Read the model definition and answer for the solid it produces. Units are mm, in the model's axes. A direction names the side the tool comes from. Give positions to 0.01 mm unless a question says otherwise; leave off trailing zeros. Write each loop counter-clockwise with the first axis right and the second up, starting at its lowest first coordinate (ties: lowest second). Pieces come first, ordered by that corner, then holes. Notation, with made-up numbers: (-32.5, 16) - (-26.5, 16) arc R32 cw to (-26.5, 46) - close; hole circle Ø7 at (-9.75, 49.5). An arc over 180 degrees is marked (long way). Answer as a JSON object with one key per item and string values. Group by question number.
```python
from build123d import *

# Parameters (mm, degrees)
SKETCH1_W           = 62.8
SKETCH1_H           = 46
SKETCH1_R           = 1.4
SKETCH1_R_2         = 15
BOSS_EXTRUDE1_DEPTH = 6
SKETCH2_W           = 8.5
SKETCH2_H           = 15
CUT_EXTRUDE1_DEPTH  = 41.459856648
FILLET1_R           = 3.1
CUT_EXTRUDE2_DEPTH  = 41.459856648


with BuildPart() as part:
    # Sketch1 → Boss-Extrude1 (new body)
    with BuildSketch(Plane(origin=(0, 0, 0), x_dir=(1, 0, 0), z_dir=(0, 1, 0))):
        with Locations((0, -1.8)):
            Rectangle(SKETCH1_W, SKETCH1_H)
        with Locations(Location((-28.3, -1.4, 0), (0, 0, 270))):
            Circle(SKETCH1_R, mode=Mode.SUBTRACT)
        with Locations(Location((28.3, 3.1, 0), (0, 0, 270))):
            Circle(SKETCH1_R, mode=Mode.SUBTRACT)
        with Locations(Location((-0.6, -0.8, 0), (0, 0, 270))):
            Circle(SKETCH1_R_2, mode=Mode.SUBTRACT)
    extrude(amount=BOSS_EXTRUDE1_DEPTH)

    # Sketch2 → Cut-Extrude1 (cut, through all)
    with BuildSketch(Plane(origin=(0, 6, 0), x_dir=(1, 0, 0), z_dir=(0, 1, 0))):
        with Locations((27.15, 13.7)):
            Rectangle(SKETCH2_W, SKETCH2_H)
        with BuildLine():
            Line((14.4, -24.8), (31.4, -24.8))
            Line((31.4, -24.8), (31.4, 0))
            Line((31.4, 0), (22.9, 0))
            ThreePointArc((22.9, 0), (20.676259907, -10.31612815), (14.4, -18.8))
            Line((14.4, -18.8), (14.4, -24.8))
        make_face()
        with BuildLine():
            Line((-17.4, -24.8), (-17.4, -16.8))
            ThreePointArc((-17.4, -16.8), (-21.820028515, -11.342696837), (-23.4, -4.5))
            Line((-23.4, -4.5), (-31.4, -4.5))
            Line((-31.4, -4.5), (-31.4, -24.8))
            Line((-31.4, -24.8), (-17.4, -24.8))
        make_face()
        with BuildLine():
            Line((-20.1, 21.2), (-20.1, 11.2))
            ThreePointArc((-20.1, 11.2), (-22.551509918, 6.728419235), (-23.4, 1.7))
            Line((-23.4, 1.7), (-31.4, 1.7))
            Line((-31.4, 1.7), (-31.4, 21.2))
            Line((-31.4, 21.2), (-20.1, 21.2))
        make_face()
    extrude(amount=-CUT_EXTRUDE1_DEPTH, mode=Mode.SUBTRACT)

    # Fillet1
    fillet1_edges = [part.edges().sort_by_distance(p)[0] for p in [
        (-31.4, 3, 4.5),
        (-31.4, 3, -1.7),
        (31.4, 3, -6.2),
        (31.4, 3, 0),
    ]]
    fillet(fillet1_edges, radius=FILLET1_R - 0.0001)  # a hair under: the kernel refuses the full size

    # Sketch3 → Cut-Extrude2 (cut, through all)
    with BuildSketch(Plane(origin=(0, 6, 0), x_dir=(1, 0, 0), z_dir=(0, 1, 0))):
        with BuildLine():
            Line((28.3, 0), (24.9, 0))
            Line((24.9, 0), (24.9, 6.2))
            Line((24.9, 6.2), (28.3, 6.2))
            ThreePointArc((28.3, 6.2), (30.492031022, 5.292031022), (31.4, 3.1))
            ThreePointArc((31.4, 3.1), (30.492031022, 0.907968978), (28.3, 0))
        make_face()
        with BuildLine():
            Line((-25.1, -4.5), (-28.3, -4.5))
            ThreePointArc((-28.3, -4.5), (-30.492031022, -3.592031022), (-31.4, -1.4))
            ThreePointArc((-31.4, -1.4), (-30.492031022, 0.792031022), (-28.3, 1.7))
            Line((-28.3, 1.7), (-25.1, 1.7))
            Line((-25.1, 1.7), (-25.1, -4.5))
        make_face()
    extrude(amount=-CUT_EXTRUDE2_DEPTH, mode=Mode.SUBTRACT)


with BuildPart() as cut_extrude2_kept_piece:
    # of the separate pieces the step leaves, the one the design keeps (cut_extrude2_pieces_kept)
    add(part.part.solids().sort_by_distance((-23.4, 0, 4.5))[0])


solid = cut_extrude2_kept_piece.part
```
1) Find section D-D, the plane x = -21. Write down the section's boundary in (y, z), and give its area (3 significant figures).
2) For a pull along Z with two mould halves and no side action, classify faces 5 (the cylindrical face through (-22.528, 3.042, -6.796)), 6 (the flat face through (11, 6, 12)), 7 (the cylindrical face through (-6.345, 2.958, 14.656)) as released by +Z, released by -Z, zero draft, split by the parting line, or undercut.
3) Find section B-B, the plane x = -0.6. Write down the section's boundary in (y, z).
4) Find the intervals of material crossed by line 1 (X direction, y = 2.4, z = 0.8); line 2 (X direction, y = 3.2, z = 3); line 3 (X direction, y = 0.35, z = -16.5), in increasing order. Write a range as [from, to].
5) Which of the six approach directions +Z, -Z, +X, -X, +Y, -Y give full straight-line access (tool end or side, diameter ignored) to faces 1 (the flat face through (-20.1, 3, -16)), 2 (the flat face through (24, 3, -6.2)), 3 (the flat face through (-24, 3, 4.5)), 4 (the flat face through (24, 3, 0))?
6) Find section C-C, the plane z = 0.8. Write down the section's boundary in (x, y).
7) Find section A-A, the plane y = 2.1. Write down the section's boundary in (x, z) (1 decimal), and give its area (3 significant figures).
8) Flat-ended cylindrical pins translate along their axes: pin 1 Ø3 at (y, z) = (2.5, 16.5) entering from +X; pin 2 Ø12 at (x, z) = (1.5, 13) entering from +Y; pin 3 Ø0.5 at (x, y) = (-24.5, 1.5) entering from +Z; pin 4 Ø3 at (y, z) = (3.5, 21) entering from +X. Find the tip coordinate at first contact, or state that the pin passes through.
Values follow:
{
 "1": {"outline": "(0, -9.93) - (6, -9.93) - (6, 12.82) - (0, 12.82) - close", "area": "136 mm2"},
 "2": {"face 5": "released by -Z", "face 6": "zero draft", "face 7": "undercut"},
 "3": {"outline": "(0, -21.2) - (6, -21.2) - (6, -14.2) - (0, -14.2) - close; (0, 15.8) - (6, 15.8) - (6, 24.8) - (0, 24.8) - close"},
 "4": {"line 1": "x = [-25.1, -15.6], [14.4, 22.89]", "line 2": "x = [-25.1, -15.44], [14.24, 22.72]", "line 3": "x = [-20.1, 22.9]"},
 "5": {"face 1": "-Z, -X, +Y, -Y", "face 2": "-Z, +X, +Y, -Y", "face 3": "+Z, -X, +Y, -Y", "face 4": "+Z, +X, +Y, -Y"},
 "6": {"outline": "(-25.1, 0) - (-15.6, 0) - (-15.6, 6) - (-25.1, 6) - close; (14.4, 0) - (22.89, 0) - (22.89, 6) - (14.4, 6) - close"},
 "7": {"outline": "(-25.1, -1.7) - (-23.4, -1.7) arc R15.3 ccw to (-20.1, -11.2) - (-20.1, -21.2) - (22.9, -21.2) - (22.9, -6.2) - (24.9, -6.2) - (24.9, 0) - (22.9, 0) arc R25 ccw to (14.4, 18.8) - (14.4, 24.8) - (-17.4, 24.8) - (-17.4, 16.8) arc R15.6 ccw to (-23.4, 4.5) - (-25.1, 4.5) - close; hole circle Ø30 at (-0.6, 0.8)", "area": "1,230 mm2"},
 "8": {"pin 1": "stops at x = 17.91", "pin 2": "stops at y = 6", "pin 3": "stops at z = 4.5", "pin 4": "stops at x = 14.4"}
}
